```python
from build123d import *

# Parameters (mm, degrees)
FLANGE_BASE1_DEPTH    = 40
ESBO_O4_R             = 6
ESBO_O4_R_2           = 8
CORTE_EXTRUS_O1_DEPTH = 1.5
FILETE1_R             = 3
CORTE_EXTRUS_O2_DEPTH = 140.396018595


# Sheet-metal steps are written as plain solids
with BuildPart() as part:
    # Esboço2 → Flange-base1 (new, symmetric)
    with BuildSketch(Plane(origin=(0, 0, 0), x_dir=(1, 0, 0), z_dir=(0, 1, 0))):
        with BuildLine():
            Line((-63, -34.5), (-63, -1.5))
            ThreePointArc((-63, -1.5), (-62.560660172, -0.439339828), (-61.5, 0))
            Line((-61.5, 0), (61.5, 0))
            ThreePointArc((61.5, 0), (62.560660172, -0.439339828), (63, -1.5))
            Line((63, -1.5), (63, -34.5))
            Line((63, -34.5), (64.5, -34.5))
            Line((64.5, -34.5), (64.5, -1.5))
            ThreePointArc((64.5, -1.5), (63.621320344, 0.621320344), (61.5, 1.5))
            Line((61.5, 1.5), (-61.5, 1.5))
            ThreePointArc((-61.5, 1.5), (-63.621320344, 0.621320344), (-64.5, -1.5))
            Line((-64.5, -1.5), (-64.5, -34.5))
            Line((-64.5, -34.5), (-63, -34.5))
        make_face()
    extrude(amount=FLANGE_BASE1_DEPTH, both=True)

    # Esboço4 → Corte-extrusão1 (cut)
    with BuildSketch(Plane(origin=(0, 0, -1.5), x_dir=(-1, 0, 0), z_dir=(0, 0, -1))):
        with Locations((44.5, 0)):
            Circle(ESBO_O4_R)
        with Locations((44.5, -20)):
            Circle(ESBO_O4_R_2)
        with Locations((44.5, 20)):
            Circle(ESBO_O4_R)
        with Locations((15, 15)):
            Circle(ESBO_O4_R_2)
        with Locations((-44.5, 0)):
            Circle(ESBO_O4_R_2)
        with Locations((-26.124574835, 18.375425165)):
            Circle(ESBO_O4_R_2)
        with Locations((-7.74914967, 0)):
            Circle(ESBO_O4_R_2)
        with Locations((-26.124574835, -18.375425165)):
            Circle(ESBO_O4_R_2)
        with Locations((15, -15)):
            Circle(ESBO_O4_R_2)
    extrude(amount=-CORTE_EXTRUS_O1_DEPTH, mode=Mode.SUBTRACT)

    # Filete1
    filete1_edges = [part.edges().sort_by_distance(p)[0] for p in [
        (63.75, -40, 34.5),
        (-63.75, -40, 34.5),
        (63.75, 40, 34.5),
        (-63.75, 40, 34.5),
    ]]
    fillet(filete1_edges, radius=FILETE1_R)

    # Esboço5 → Corte-extrusão2 (cut, through all)
    with BuildSketch(Plane.ZY.offset(64.5)):
        with BuildLine():
            Line((18.3, 33.75), (21.3, 33.75))
            ThreePointArc((21.3, 33.75), (23.05, 32), (21.3, 30.25))
            Line((21.3, 30.25), (18.3, 30.25))
            ThreePointArc((18.3, 30.25), (16.55, 32), (18.3, 33.75))
        make_face()
        with BuildLine():
            Line((18.3, -30.25), (21.3, -30.25))
            ThreePointArc((21.3, -30.25), (23.05, -32), (21.3, -33.75))
            Line((21.3, -33.75), (18.3, -33.75))
            ThreePointArc((18.3, -33.75), (16.55, -32), (18.3, -30.25))
        make_face()
    extrude(amount=-CORTE_EXTRUS_O2_DEPTH, mode=Mode.SUBTRACT)


solid = part.part
```
Check sheet for the modelled part. Datum: model origin and axes. Units: mm. A direction names the side the tool comes from. Give positions to 0.01 mm unless a question says otherwise; leave off trailing zeros. Order: outer loops, then holes, each group sorted by start corner. A loop starts at its lowest first (then second) coordinate and runs counter-clockwise, first axis right, second up. Notation, with made-up numbers: M 74,-8 L 89,-8 A28 ccw 89,23 Z; hole C 14.5,20.5 d2. An arc over 180 degrees is marked long. Answer in a Markdown table with one row per item.
1) Cross-section at C-C, the plane y = 32. Enter the section's corners in (x, z), plus the area to 3 significant figures.
Filled sheet:
| item | result |
|---|---|
| outline | M -64.5,1.5 A3 ccw -61.5,-1.5 L 61.5,-1.5 A3 ccw 64.5,1.5 L 64.5,16.55 L 63,16.55 L 63,1.5 A1.5 cw 61.5,0 L -61.5,0 A1.5 cw -63,1.5 L -63,16.55 L -64.5,16.55 Z; M -64.5,23.05 L -63,23.05 L -63,34.5 L -64.5,34.5 Z; M 63,23.05 L 64.5,23.05 L 64.5,34.5 L 63,34.5 Z |
| area | 275 mm2 |
2) Thickness scan on L1, parallel to Y at x = -15, z = -1.1; L2, parallel to Y at x = -44.5, z = -1; L3, parallel to X at y = -20, z = 3. Record the ranges inside material, lowest first. Write a range as [from, to].
Filled sheet:
| item | result |
|---|---|
| L1 | y = [-40, -23], [-7, 7], [23, 40] |
| L2 | y = [-40, -28], [-12, -6], [6, 14], [26, 40] |
| L3 | x = [-64.5, -63], [63, 64.5] |
3) Release check for a two-part mould opening along Y. For faces 3 (the cylindrical face through (63.76, -39.14, 33.6)), 4 (the cylindrical face through (50.849, -4.868, -0.76)), 5 (the cylindrical face through (63.64, 0.56, -0.6)), 6 (the cylindrical face through (-38.506, 20.264, -0.76)) record: +Y half, -Y half, draft (parallel to the pull), parting line (faces both ways), or undercut.
Filled sheet:
| item | result |
|---|---|
| face 3 | -Y half |
| face 4 | undercut |
| face 5 | draft |
| face 6 | undercut |
4) Access from +Z, -Z, +X, -X, +Y, -Y to the whole of each face (thin tool, end or side, straight path). Record for faces 1 (the flat face through (63, 1, 18)), 2 (the cylindrical face through (63.76, 39.14, 33.6)).
Filled sheet:
| item | result |
|---|---|
| face 1 | +Z, +Y, -Y |
| face 2 | +Z, +X, -X, +Y |
5) Cross-section at B-B, the plane z = 26.5. Enter the section's corners in (x, y), plus the area to 3 significant figures.
Filled sheet:
| item | result |
|---|---|
| outline | M -64.5,-40 L -63,-40 L -63,40 L -64.5,40 Z; M 63,-40 L 64.5,-40 L 64.5,40 L 63,40 Z |
| area | 240 mm2 |
6) Gauge pin test, flat ends, axial feed: P1, Ø18.5, axis at x = -44.5, y = -20, coming from the +Z side; P2, Ø18.5, axis at x = 7.75, y = 0, coming from the -Z side. Record the tip position at first contact, or that the pin passes through.
Filled sheet:
| item | result |
|---|---|
| P1 | stops at z = 0 |
| P2 | stops at z = -1.5 |
7) Cross-section at A-A, the plane x = -15. Enter the section's corners in (y, z), plus the area to 3 significant figures.
Filled sheet:
| item | result |
|---|---|
| outline | M -40,-1.5 L -23,-1.5 L -23,0 L -40,0 Z; M -7,-1.5 L 7,-1.5 L 7,0 L -7,0 Z; M 23,-1.5 L 40,-1.5 L 40,0 L 23,0 Z |
| area | 72.0 mm2 |
8) Cross-section at D-D, the plane x = 44.5. Enter the section's corners in (y, z), plus the area to 3 significant figures.
Filled sheet:
| item | result |
|---|---|
| outline | M -40,-1.5 L -8,-1.5 L -8,0 L -40,0 Z; M 8,-1.5 L 40,-1.5 L 40,0 L 8,0 Z |
| area | 96.0 mm2 |
